Check sheet for the modelled part. Datum: model origin and axes. Units: mm. Face numbers are marked on the shaded views. A direction names the side the tool comes from. Give positions to 0.01 mm unless a question says otherwise; leave off trailing zeros. Loops run counter-clockwise (first coordinate to the right, second up) from the corner with the lowest first, then second, coordinate; pieces in that order, holes last. Notation, with made-up numbers: (79.25, 51.5) - (132.25, 51.5) arc R27 cw to (132.25, 89.5) - close; hole circle Ø9 at (-28.5, -28.5). An arc over 180 degrees is marked (long way). Use CSV: the item, a comma, the result in double quotes.
from build123d import *

# Parameters (mm, degrees)
BOSS_EXTRUDE1_DEPTH = 35
CUT_EXTRUDE1_REACH  = 160.215
SKETCH3_R           = 5
SKETCH4_R           = 10.5
CUT_EXTRUDE2_DEPTH  = 10
FILLET1_R           = 8


with BuildPart() as part:
    # Sketch2 → Boss-Extrude1 (new body)
    with BuildSketch(Plane(origin=(0, 0, 0), x_dir=(0, 0, -1), z_dir=(1, 0, 0))):
        with BuildLine():
            Line((-27.24, -11), (-54.920224718, -11))
            Line((-54.920224718, -11), (-54.920224718, 0))
            Line((-54.920224718, 0), (-54.920224718, 13.24))
            Line((-54.920224718, 13.24), (-16.24, 13.24))
            Line((-16.24, 13.24), (-16.24, 0))
            ThreePointArc((-16.24, 0), (0, -16.24), (16.24, 0))
            Line((16.24, 0), (16.24, 13.24))
            Line((16.24, 13.24), (78.76, 13.24))
            Line((78.76, 13.24), (78.76, 0))
            ThreePointArc((78.76, 0), (95, -16.24), (111.24, 0))
            Line((111.24, 0), (111.24, 13.24))
            Line((111.24, 13.24), (149.920224718, 13.24))
            Line((149.920224718, 13.24), (149.920224718, 0))
            Line((149.920224718, 0), (149.920224718, -11))
            Line((149.920224718, -11), (122.24, -11))
            ThreePointArc((122.24, -11), (95, -23.24), (67.76, -11))
            Line((67.76, -11), (27.24, -11))
            ThreePointArc((27.24, -11), (0, -23.24), (-27.24, -11))
        make_face()
    extrude(amount=BOSS_EXTRUDE1_DEPTH)

    # Sketch3 → Cut-Extrude1 (cut, up to next)
    with BuildSketch(Plane(origin=(0, 13.24, 0), x_dir=(1, 0, 0), z_dir=(0, 1, 0)), mode=Mode.PRIVATE) as cut_extrude1_sk1:
        with Locations(Location((17.5, -41.080112359, 0), (0, 0, 270))):
            Circle(SKETCH3_R)
    cut_extrude1_tool1 = extrude(cut_extrude1_sk1.sketch, amount=-CUT_EXTRUDE1_REACH, mode=Mode.PRIVATE) & part.part
    # Sketch3 → Cut-Extrude1 (cut, up to next)
    with BuildSketch(Plane(origin=(0, 13.24, 0), x_dir=(1, 0, 0), z_dir=(0, 1, 0)), mode=Mode.PRIVATE) as cut_extrude1_sk2:
        with Locations(Location((17.5, 136.080112359, 0), (0, 0, 270))):
            Circle(SKETCH3_R)
    cut_extrude1_tool2 = extrude(cut_extrude1_sk2.sketch, amount=-CUT_EXTRUDE1_REACH, mode=Mode.PRIVATE) & part.part
    # Sketch3 → Cut-Extrude1 (cut, up to next)
    with BuildSketch(Plane(origin=(0, 13.24, 0), x_dir=(1, 0, 0), z_dir=(0, 1, 0)), mode=Mode.PRIVATE) as cut_extrude1_sk3:
        with Locations(Location((17.5, 47.5, 0), (0, 0, 270))):
            Circle(SKETCH3_R)
    cut_extrude1_tool3 = extrude(cut_extrude1_sk3.sketch, amount=-CUT_EXTRUDE1_REACH, mode=Mode.PRIVATE) & part.part
    add(cut_extrude1_tool1.solids().sort_by_distance((17.5, 13.24, 41.080112))[0], mode=Mode.SUBTRACT)
    add(cut_extrude1_tool2.solids().sort_by_distance((17.5, 13.24, -136.080112))[0], mode=Mode.SUBTRACT)
    add(cut_extrude1_tool3.solids().sort_by_distance((17.5, 13.24, -47.5))[0], mode=Mode.SUBTRACT)

    # Sketch4 → Cut-Extrude2 (cut)
    with BuildSketch(Plane.XZ.offset(11)):
        with Locations(Location((17.5, -47.5, 0), (0, 0, 270))):
            Circle(SKETCH4_R)
        with Locations(Location((17.5, -136.080112359, 0), (0, 0, 270))):
            Circle(SKETCH4_R)
        with Locations(Location((17.5, 41.080112359, 0), (0, 0, 270))):
            Circle(SKETCH4_R)
    extrude(amount=-CUT_EXTRUDE2_DEPTH, mode=Mode.SUBTRACT)

    # Fillet1
    fillet1_edges = [part.edges().sort_by_distance(p)[0] for p in [
        (35, 1.12, 54.920224718),
        (0, 1.12, -149.920224718),
        (0, 1.12, 54.920224718),
        (35, 1.12, -149.920224718),
    ]]
    fillet(fillet1_edges, radius=FILLET1_R)


solid = part.part
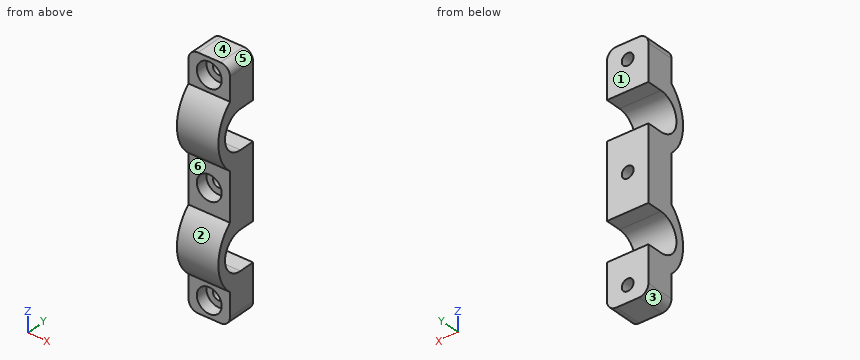
1. Release check for a two-part mould opening along Z. For the marked faces 1, 2, 3 and 4 record: released by +Z, released by -Z, zero draft, split by the parting line, or undercut.
Completed:
face 1,"zero draft"
face 2,"undercut"
face 3,"released by -Z"
face 4,"released by +Z"
2. Sectioned sample at D-D, the plane x = 15. State how many separate pieces and enclosed holes the cut face has, and give its area (3 significant figures).
Completed:
separate pieces,"4"
enclosed holes,"0"
area,"3,220 mm²"
3. Sectioned sample at C-C, the plane x = 24.5. Record the boundary of the cut face in (y, z).
Completed:
outline,"(-11, -149.92) - (13.24, -149.92) - (13.24, -111.24) - (0, -111.24) arc R16.24 cw to (0, -78.76) - (13.24, -78.76) - (13.24, -16.24) - (0, -16.24) arc R16.24 cw to (0, 16.24) - (13.24, 16.24) - (13.24, 54.92) - (-11, 54.92) - (-11, 48.91) - (-1, 48.91) - (-1, 33.25) - (-11, 33.25) - (-11, 27.24) arc R36.43 ccw to (-11, -27.24) - (-11, -39.67) - (-1, -39.67) - (-1, -55.33) - (-11, -55.33) - (-11, -67.76) arc R36.43 ccw to (-11, -122.24) - (-11, -128.25) - (-1, -128.25) - (-1, -143.91) - (-11, -143.91) - close"
4. Scan lines: line 1 along Z through (x, y) = (10, 11.5); line 2 along Z through (x, y) = (18, 5); line 3 along X through (y, z) = (9.5, 41.5). Record each from-to range of solid material in increasing order.
Completed:
line 1,"z = -149.92 to -111.24, -78.76 to -16.24, 16.24 to 54.92"
line 2,"z = -149.92 to -141.06, -131.11 to -111.24, -78.76 to -52.47, -42.53 to -16.24, 16.24 to 36.11, 46.06 to 54.92"
line 3,"x = 0 to 12.52, 22.48 to 35"
5. Sectioned sample at B-B, the plane z = -47.5. Record the boundary of the cut face in (x, y), and give its area (3 significant figures).
Completed:
outline,"(0, -11) - (7, -11) - (7, -1) - (12.5, -1) - (12.5, 13.24) - (0, 13.24) - close; (22.5, -1) - (28, -1) - (28, -11) - (35, -11) - (35, 13.24) - (22.5, 13.24) - close"
area,"496 mm²"
6. Go/stop test with flat-tipped pins: pin 1 Ø17 at (x, z) = (20.5, -133) entering from -Y; pin 2 Ø13 at (x, z) = (17.5, 41.08) entering from -Y; pin 3 Ø6 at (x, z) = (26, -2.5) entering from -Y. Record where each tip stops, or that it passes through.
Completed:
pin 1,"stops at y = -11"
pin 2,"stops at y = -1"
pin 3,"stops at y = -23.24"
7. Sectioned sample at A-A, the plane y = 3.5. Record the boundary of the cut face in (x, z), and give its area (3 significant figures).
Completed:
outline,"(0, -141.92) arc R8 ccw to (8, -149.92) - (27, -149.92) arc R8 ccw to (35, -141.92) - (35, -111.24) - (0, -111.24) - close; (0, -78.76) - (35, -78.76) - (35, -16.24) - (0, -16.24) - close; (0, 16.24) - (35, 16.24) - (35, 46.92) arc R8 ccw to (27, 54.92) - (8, 54.92) arc R8 ccw to (0, 46.92) - close; hole circle Ø10 at (17.5, -136.08); hole circle Ø10 at (17.5, -47.5); hole circle Ø10 at (17.5, 41.08)"
area,"4,610 mm²"
8. Set-up check for the marked faces 5 and 6: record each of +Z, -Z, +X, -X, +Y, -Y from which the full face is reachable in a straight line by a thin tool's end or side.
Completed:
face 5,"+Z, +X, +Y, -Y"
face 6,"+X, -X, -Y"
